Geometry: final body of the model. Coordinates: model frame, mm. Give positions to 0.01 mm unless a question says otherwise; leave off trailing zeros. Write each loop counter-clockwise with the first axis right and the second up, starting at its lowest first coordinate (ties: lowest second). Pieces come first, ordered by that corner, then holes. Notation, with made-up numbers: (51.5, 67) - (108.5, 67) arc R28 ccw to (108.5, 89) - close; hole circle Ø1 at (-31.75, -37). An arc over 180 degrees is marked (long way). Use CSV: the item, a comma, the result in double quotes. Start each with the question number.
(1) First-contact query: pin 1 Ø1.5 at (x, y) = (1.5, 1) entering from +Z; pin 2 Ø1.5 at (x, y) = (7, 1.5) entering from +Z; pin 3 Ø1.5 at (y, z) = (1.5, 8.5) entering from +X. Flat tips, straight axial feed; report the tip coordinate or a pass-through.
(2) Section B-B on x = 8. Output: boundary loops of the cut face in (y, z), and give its area (3 significant figures).
(3) Section C-C on z = 8.5. Output: boundary loops of the cut face in (x, y), and give its area (3 significant figures).
(4) Section A-A on y = 0.95. Output: boundary loops of the cut face in (x, z), and give its area (3 significant figures).
(5) Draft query along X for faces 1 (the cylindrical face through (3, 3, 1)), 2 (the flat face through (0, 3, 4.5)), 3 (the flat face through (5, 3, 5)), 4 (the flat face through (3, 0, 3)). Return one class per face: released by +X, released by -X, zero draft, split by the parting line, or undercut.
(6) Line query: probe 1 along X at (y, z) = (3.45, 9); probe 2 along X at (y, z) = (4.3, 3). Output: solid intervals per line, ascending. Write a range as [from, to].
from build123d import *

# Parameters (mm, degrees)
BOSS_EXTRUDE1_DEPTH = 6
SKETCH2_R           = 1
CUT_EXTRUDE1_DEPTH  = 16.362291496


with BuildPart() as part:
    # Sketch1 → Boss-Extrude1 (new body)
    with BuildSketch(Plane(origin=(0, 0, 0), x_dir=(1, 0, 0), z_dir=(0, 1, 0))):
        Polygon((0, 0), (10, 0), (0, -10), align=None)
    extrude(amount=BOSS_EXTRUDE1_DEPTH)

    # Sketch2 → Cut-Extrude1 (cut, through all)
    with BuildSketch(Plane(origin=(0, 6, 0), x_dir=(1, 0, 0), z_dir=(0, 1, 0))):
        with Locations((0, -6)):
            Circle(SKETCH2_R)
        with Locations((0, -3)):
            Circle(SKETCH2_R)
        with Locations((3, 0)):
            Circle(SKETCH2_R)
        with Locations((6, 0)):
            Circle(SKETCH2_R)
    extrude(amount=-CUT_EXTRUDE1_DEPTH, mode=Mode.SUBTRACT)


solid = part.part
Check values:
1,pin 1,"stops at z = 9.25"
1,pin 2,"stops at z = 3.75"
1,pin 3,"stops at x = 2.25"
2,outline,"(0, 0) - (6, 0) - (6, 2) - (0, 2) - close"
2,area,"12.0 mm²"
3,outline,"(0, 0) - (1.5, 0) - (1.5, 6) - (0, 6) - close"
3,area,"9.00 mm²"
4,outline,"(0, 0) - (2, 0) arc R1 cw to (4, 0) - (5, 0) arc R1 cw to (7, 0) - (10, 0) - (0, 10) - (0, 7) arc R1 cw to (0, 5) - (0, 4) arc R1 cw to (0, 2) - close"
4,area,"43.7 mm²"
5,face 1,"undercut"
5,face 2,"released by -X"
5,face 3,"released by +X"
5,face 4,"zero draft"
6,probe 1,"x = [0, 1]"
6,probe 2,"x = [1, 7]"
